from build123d import *

# Parameters (mm, degrees)
BLANKSKE_W              = 151
BLANKSKE_H              = 11.5
BLANK_DEPTH             = 5
TOOTHCUTSIM_DEPTH       = 152.519800686
TEETHCUTS_COUNT         = 33
TEETHCUTS_PITCH         = 4.712388975
CROQUIS1_W              = 70
CROQUIS1_H              = 8.125
SALIENTE_EXTRUIR1_DEPTH = 5


with BuildPart() as part:
    # BlankSke → Blank (new body)
    with BuildSketch(Plane.XY):
        with Locations((75.5, 5.75)):
            Rectangle(BLANKSKE_W, BLANKSKE_H)
    extrude(amount=-BLANK_DEPTH)

    # TooCutSkeSim → ToothCutSim (cut, through all)
    with BuildSketch(Plane.XY):
        Polygon((0.654653055, 8.125), (-0.654653055, 8.125), (-1.892297439, 11.5254), (1.892297439, 11.5254), align=None)
    toothcutsim = extrude(amount=-TOOTHCUTSIM_DEPTH, mode=Mode.SUBTRACT)

    # TeethCuts: ToothCutSim ×33
    with Locations(*[(i * TEETHCUTS_PITCH, 0, 0) for i in range(1, TEETHCUTS_COUNT)]):
        add(toothcutsim, mode=Mode.SUBTRACT)

    # Croquis1 → Saliente-Extruir1 (add)
    with BuildSketch(Plane(origin=(151, 0, 0), x_dir=(0, 0, -1), z_dir=(1, 0, 0))):
        with Locations((2.5, 4.0625)):
            Rectangle(CROQUIS1_W, CROQUIS1_H)
    extrude(amount=SALIENTE_EXTRUIR1_DEPTH)


solid = part.part
Part model, mm, in its own coordinate system. Coordinates: 2 decimals unless noted, no trailing zeros. Loops run counter-clockwise (first coordinate to the right, second up) from the corner with the lowest first, then second, coordinate; pieces in that order, holes last. Notation, with made-up numbers: M 25.5,20 L 60.5,20 A16 ccw 60.5,45 Z; hole C 44,46.5 d3. An arc over 180 degrees is marked long. Use a Markdown table: item, result. Add a question column.
Q1. Probe L1, parallel to X at y = 8, z = -10.5; L2, parallel to Z at x = 96.5, y = 5.5. List the from-to ranges inside material, lowest first.
Q2. Pin check, flat tips, straight feed: P1, Ø5, axis at x = 65.5, y = 3, coming from the -Z side; P2, Ø1.5, axis at y = 2.5, z = -9, coming from the -X side; P3, Ø0.7, axis at x = 132, z = -2.5, coming from the +Y side (3 decimals). Stop position of each tip, or through.
Q3. Cut at A-A (y = 1.75). Write the cut outline in (x, z).
Q4. Cut at B-B (z = -23). Write the cut outline in (x, y) (3 decimals), and give its area (3 significant figures).
Q5. Mould opens along X. For faces 1 (the flat face through (24.84, 9.84, -2.46)), 2 (the flat face through (1.28, 9.84, -2.46)) say: +X half, -X half, draft (parallel to the pull), parting line (faces both ways), or undercut.
Worked out:
| question | item | result |
|---|---|---|
| 1 | L1 | x = 151 to 156 |
| 1 | L2 | z = -5 to 0 |
| 2 | P1 | stops at z = -5 |
| 2 | P2 | stops at x = 151 |
| 2 | P3 | stops at y = 8.125 |
| 3 | outline | M 0,-5 L 151,-5 L 151,-37.5 L 156,-37.5 L 156,32.5 L 151,32.5 L 151,0 L 0,0 Z |
| 4 | outline | M 151,0 L 156,0 L 156,8.125 L 151,8.125 Z |
| 4 | area | 40.6 mm2 |
| 5 | face 1 | undercut |
| 5 | face 2 | -X half |
